```python
from build123d import *

# Parameters (mm, degrees)
LPATTERN1_COUNT = 2
LPATTERN1_PITCH = 1.524


with BuildPart() as part:
    # Sketch1 → Revolve1 (revolve)
    with BuildSketch(Plane.XY, mode=Mode.PRIVATE) as revolve1_sk:
        Polygon((9.4615, 0.762), (9.4615, 56.388), (8.6995, 57.15), (0, 57.15), (0, 2.286), (4.5466, 2.286), (4.8006, 2.032), (4.8006, 0), (8.6995, 0), align=None)
    revolve(revolve1_sk.sketch.rotate(Axis((0, 0, 0), (0, 1, 0)), 90), axis=Axis((0, 0, 0), (0, 1, 0)))  # turned: the seam where the file's is

    # Sketch2 → Cut-Revolve1 (revolve, cut)
    with BuildSketch(Plane.XY, mode=Mode.PRIVATE) as cut_revolve1_sk:
        with BuildLine():
            Line((9.525, 36.2585), (9.525, 36.8935))
            Line((9.525, 36.8935), (9.387105122, 36.755605122))
            ThreePointArc((9.387105122, 36.755605122), (9.312710245, 36.576), (9.387105122, 36.396394878))
            Line((9.387105122, 36.396394878), (9.525, 36.2585))
        make_face()
    cut_revolve1 = revolve(cut_revolve1_sk.sketch.rotate(Axis((0, 0, 0), (0, 1, 0)), 90), axis=Axis((0, 0, 0), (0, 1, 0)), mode=Mode.SUBTRACT)  # turned: the seam where the file's is

    # LPattern1: Cut-Revolve1 ×2
    with Locations(*[(0, i * LPATTERN1_PITCH, 0) for i in range(1, LPATTERN1_COUNT)]):
        add(cut_revolve1, mode=Mode.SUBTRACT)


solid = part.part
```
Here's how the part is built. I have some questions about the finished solid (model axes, mm). A direction names the side the tool comes from. Give positions to 0.01 mm unless a question says otherwise; leave off trailing zeros. Loops run counter-clockwise (first coordinate to the right, second up) from the corner with the lowest first, then second, coordinate; pieces in that order, holes last. Notation, with made-up numbers: (1.5, -35) -> (40.5, -35) arc R14 ccw to (40.5, -10) -> close; hole circle Ø3 at (58, 14). An arc over 180 degrees is marked (long way). Use one line per item in the form item = value. Start each with the question number.
1) Please list where these lines run through material, in increasing order: line 1 along X through (y, z) = (1.3, 0); line 2 along Y through (x, z) = (0.5, 3); line 3 along X through (y, z) = (0.6, 0).
2) Which directions (+Z, -Z, +X, -X, +Y, -Y) give clear straight access to the entire face, cutting with the end or side of a thin tool? Please do faces 1 (the face through (-4.76, 1, 0.62)), 2 (the face through (0, 57.15, 0)).
3) For P1, Ø2.5, axis at x = 2, z = 0, coming from the -Y side; P2, Ø3, axis at x = 3, z = -1, coming from the -Y side; P3, Ø2, axis at x = -2, y = 37.5, coming from the -Z side, each with a flat end and sliding along its axis, tell me the tip position at first contact or that it passes through.
4) Imagine slicing it at C-C (y = 53). Please give me the cut outline in (x, z), then the cut area to 3 significant figures.
Check values:
q1.line_1 = -9.46 to -4.8, 4.8 to 9.46
q1.line_2 = 2.29 to 57.15
q1.line_3 = -9.3 to -4.8, 4.8 to 9.3
q2.face_1 = -Y
q2.face_2 = +Z, -Z, +X, -X, +Y
q3.P1 = 2.29
q3.P2 = 2.17
q3.P3 = -9.41
q4.outline = circle Ø18.92 at (0, 0)
q4.area = 281 mm^2
